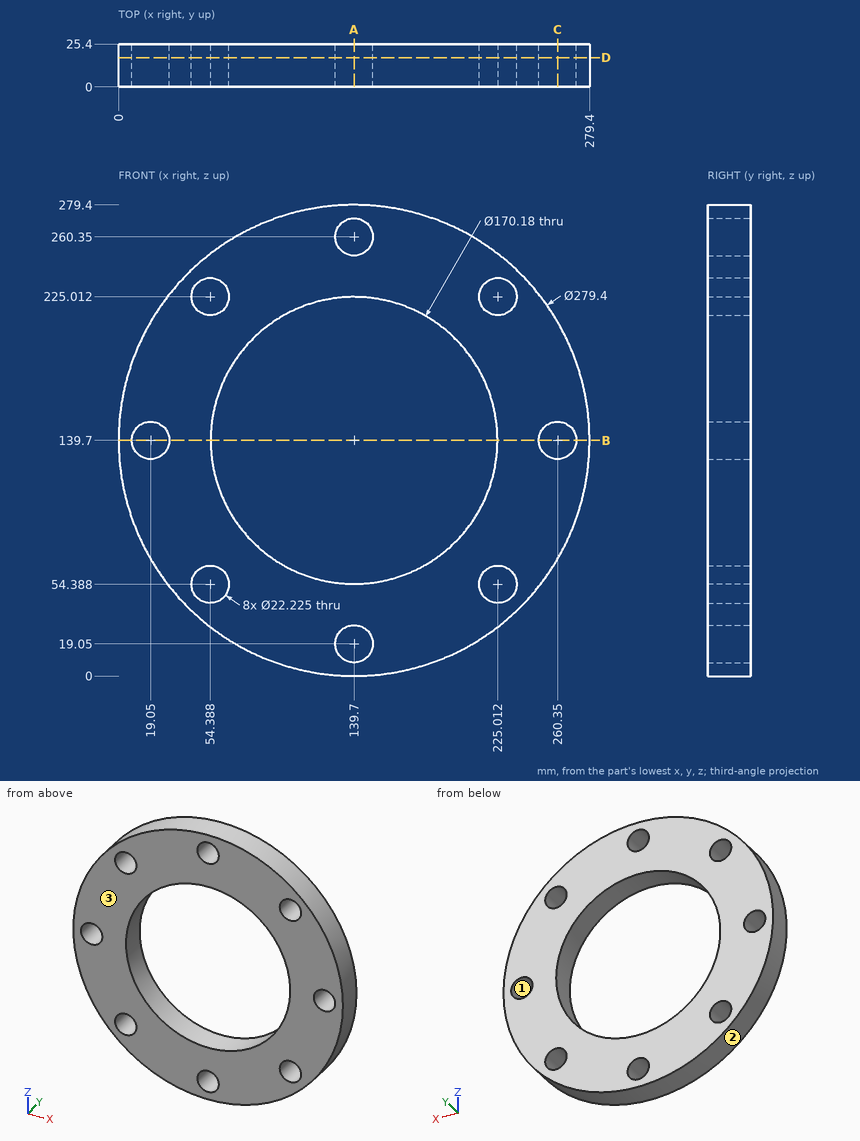
The drawing under review shows one solid part. Ordinate dimensions are in mm from its lowest x, y, z. Round coordinates to 2 decimals unless told otherwise and drop trailing zeros. Write each loop counter-clockwise with the first axis right and the second up, starting at its lowest first coordinate (ties: lowest second). Pieces come first, ordered by that corner, then holes.
(1) Mouldability with a two-part tool opening along X and no side actions: class the marked faces 1, 2 and 3 as +X half, -X half, draft (parallel to the pull), parting line (faces both ways), or undercut.
(2) We need section B-B on z = 139.7. Give the boundary of the cut face in (x, y), and give its area (4 significant figures).
(3) We need section A-A on x = 139.7. Give the boundary of the cut face in (y, z), and give its area (4 significant figures).
(4) We need section D-D on y = 17.25. Give the number of separate pieces and of enclosed holes in the cut face, and give its area (3 significant figures).
(5) Insertion check: pin 1 (1 mm diameter, centred on x = 71.5, y = 6, fed in from -Z); pin 2 (8 mm diameter, centred on y = 16.5, z = 128.5, fed in from -X); pin 3 (18 mm diameter, centred on x = 225.01, z = 54.39, fed in from -Y); pin 4 (6 mm diameter, centred on y = 22.5, z = 151.5, fed in from -X). Each pin has a flat end and moves straight along its axis. Give the tip position at first contact, or say it passes through.
(6) We need section C-C on x = 260.35. Give the boundary of the cut face in (y, z) (1 decimal).
(7) Wall thickness on L1, parallel to X at y = 2.75, z = 141 (1 decimal); L2, parallel to Z at x = 139.7, y = 16.75; L3, parallel to X at y = 6, z = 228.5 (1 decimal): over which ranges is each line inside the solid? List them lowest first.
Findings below:
1. face 1: undercut
1. face 2: parting line
1. face 3: draft
2. outline: (0, 0) - (7.94, 0) - (7.94, 25.4) - (0, 25.4) - close; (30.16, 0) - (54.61, 0) - (54.61, 25.4) - (30.16, 25.4) - close; (224.79, 0) - (249.24, 0) - (249.24, 25.4) - (224.79, 25.4) - close; (271.46, 0) - (279.4, 0) - (279.4, 25.4) - (271.46, 25.4) - close
2. area: 1,645 mm2
3. outline: (0, 0) - (25.4, 0) - (25.4, 7.94) - (0, 7.94) - close; (0, 30.16) - (25.4, 30.16) - (25.4, 54.61) - (0, 54.61) - close; (0, 224.79) - (25.4, 224.79) - (25.4, 249.24) - (0, 249.24) - close; (0, 271.46) - (25.4, 271.46) - (25.4, 279.4) - (0, 279.4) - close
3. area: 1,645 mm2
4. separate pieces: 1
4. enclosed holes: 9
4. area: 35,500 mm2
5. pin 1: stops at z = 17.5
5. pin 2: stops at x = 0.19
5. pin 3: passes through
5. pin 4: stops at x = 0.28
6. outline: (0, 69.3) - (25.4, 69.3) - (25.4, 128.6) - (0, 128.6) - close; (0, 150.8) - (25.4, 150.8) - (25.4, 210.1) - (0, 210.1) - close
7. L1: x = 0 to 8, 30.1 to 54.6, 224.8 to 249.3, 271.4 to 279.4
7. L2: z = 0 to 7.94, 30.16 to 54.61, 224.79 to 249.24, 271.46 to 279.4
7. L3: x = 31.9 to 43.8, 64.9 to 214.5, 235.6 to 247.5
